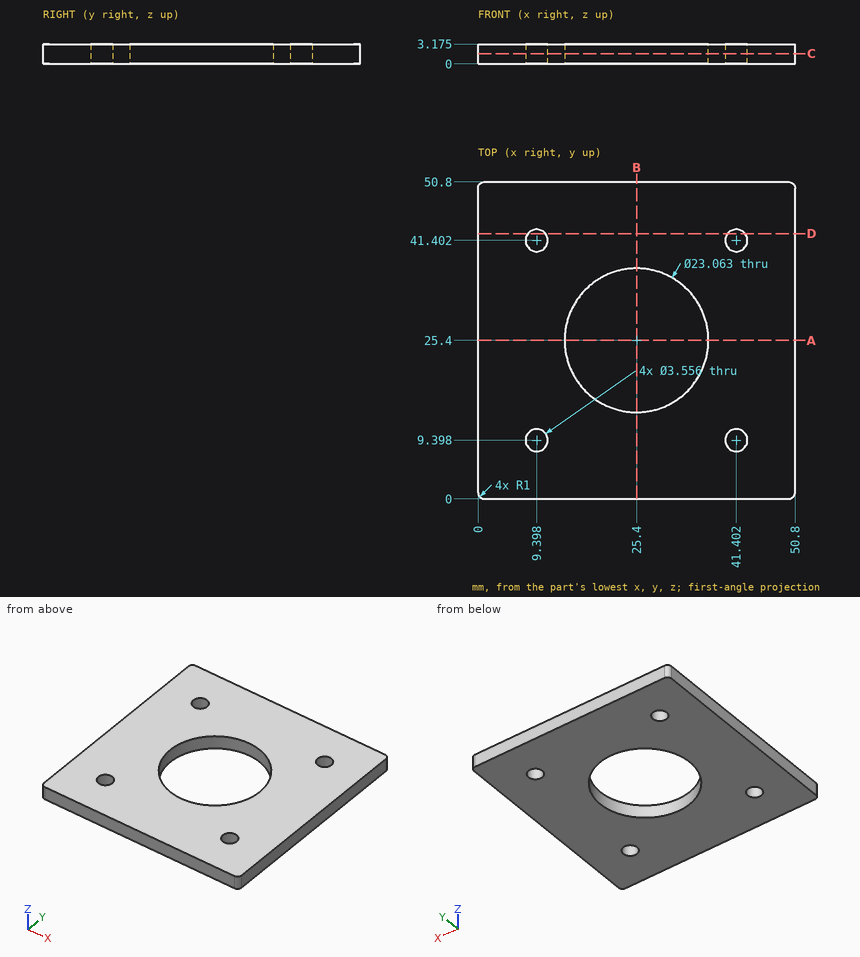
Job drawing, mm, ordinate dimensions from the low corner. One solid piece. Give positions to 0.01 mm unless a question says otherwise; leave off trailing zeros. Order: outer loops, then holes, each group sorted by start corner. A loop starts at its lowest first (then second) coordinate and runs counter-clockwise, first axis right, second up. Notation, with made-up numbers: M 45.5,-4.75 L 96.5,-4.75 A34 ccw 96.5,31.25 Z; hole C -26.75,46 d8. An arc over 180 degrees is marked long. Put each result on its own line as item: value. Start each with the question number.
(1) Drill centre lines: L1, parallel to X at y = 43, z = 2.05; L2, parallel to Y at x = 41, z = 1.25; L3, parallel to Y at x = 25.4, z = 1.7. Where is each one in solid material? Low to high. Write a range as [from, to].
(2) Band-saw the part on D-D on y = 42.5. Give the cut face in (x, z) (1 decimal).
(3) Band-saw the part on C-C on z = 1.65. Give the cut face in (x, y).
(4) Band-saw the part on A-A on y = 25.4. Give the cut face in (x, z) (1 decimal).
Results below:
1. L1: x = [0, 8.62], [10.18, 40.62], [42.18, 50.8]
1. L2: y = [0, 7.67], [11.13, 39.67], [43.13, 50.8]
1. L3: y = [0, 13.87], [36.93, 50.8]
2. outline: M 0,0 L 8,0 L 8,3.2 L 0,3.2 Z; M 10.8,0 L 40,0 L 40,3.2 L 10.8,3.2 Z; M 42.8,0 L 50.8,0 L 50.8,3.2 L 42.8,3.2 Z
3. outline: M 0,1 A1 ccw 1,0 L 49.8,0 A1 ccw 50.8,1 L 50.8,49.8 A1 ccw 49.8,50.8 L 1,50.8 A1 ccw 0,49.8 Z; hole C 9.4,9.4 d3.56; hole C 9.4,41.4 d3.56; hole C 25.4,25.4 d23.06; hole C 41.4,9.4 d3.56; hole C 41.4,41.4 d3.56
4. outline: M 0,0 L 13.9,0 L 13.9,3.2 L 0,3.2 Z; M 36.9,0 L 50.8,0 L 50.8,3.2 L 36.9,3.2 Z
